Autodesk Inventor part; units mm, degrees
ref_plane "Work Plane1" through (0, -4, 0) normal (1, 0, 0) x (0, 0, -1)
ref_plane "YZ Plane" through (0, 0, 0) normal (1, 0, 0) x (0, 1, 0)
ref_plane "XZ Plane" through (0, 0, 0) normal (0, 1, 0) x (-1, 0, 0)
sketch "Sketch1" plane through (0, 0, 0) normal (0, 0, 1) x (1, 0, 0)
  line L0 (-15, -4) -> (15, -4)
  line L1 (15, -4) -> (15, 4)
  line L2 (15, 4) -> (-15, 4)
  line L3 (-15, 4) -> (-15, -4)
  line L4 (-15, -4) -> (15, 4) construction
  line L5 (15, -4) -> (-15, 4) construction
  point P0 (0, 0)
  dimension "d2" = 30
  dimension "d3" = 8
extrude "Extrusion1" add sketch "Sketch1" against normal blind 40
sketch "Sketch2" plane through (0, 0, 0) normal (0, 0, 1) x (1, 0, 0)
  circle A0 centre (0, 1.5) radius 2.75
  line L0 (-15, -4) -> (15, -4)
  point P0 (0, 0)
  point P1 (-9, -4)
  point P2 (9, -4)
  dimension "d7" = 5.5
  dimension "d8" = 5.5
extrude "Extrusion2" cut sketch "Sketch2" against normal blind 40
sketch "Sketch3" plane through (15, 4, 0) normal (0, 1, 0) x (1, 0, 0)
  circle A0 centre (-6, 8) radius 2
  line L0 (0, 0) -> (0, 40)
  line L1 (0, 0) -> (-13.8544, 0)
  point P0 (-15, 0)
  dimension "d11" = 4
  dimension "d12" = 6
  dimension "d13" = 8
extrude "Extrusion3" cut sketch "Sketch3" against normal blind 40
pattern_linear "Rectangular Pattern1" count 2 spacing 23 along (0, 0, -1) of "Extrusion3"
ref_plane "Work Plane1" through (0, -4, 0) normal (1, 0, 0) x (0, 0, -1)
mirror "Mirror1" about plane through (0, -4, 0) normal (1, 0, 0) of "Extrusion3", "Rectangular Pattern1"
properties part number "Differential_drive_wheel"
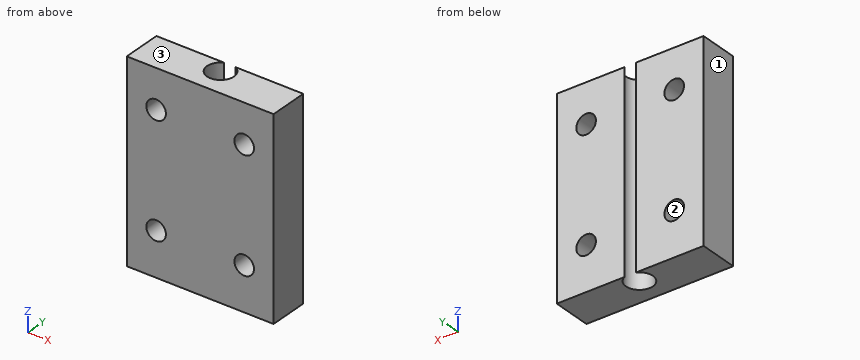
Build history of the part. All positions in model axes, mm. Face numbers are marked on the shaded views. Give positions to 0.01 mm unless a question says otherwise; leave off trailing zeros. Loops run counter-clockwise (first coordinate to the right, second up) from the corner with the lowest first, then second, coordinate; pieces in that order, holes last.
1) Band-saw the part on B-B on y = 1.5. List the corners of the cut face in (x, z).
Values follow:
outline: (-15, -40) - (-2.75, -40) - (-2.75, 0) - (-15, 0) - close; (2.75, -40) - (15, -40) - (15, 0) - (2.75, 0) - close; hole circle Ø4 at (-9, -31); hole circle Ø4 at (-9, -8); hole circle Ø4 at (9, -31); hole circle Ø4 at (9, -8)
2) Band-saw the part on D-D on z = -17. List the corners of the cut face in (x, y), then the cut area to 3 significant figures.
Values follow:
outline: (-15, -4) - (15, -4) - (15, 4) - (1.15, 4) arc R2.75 cw (long way) to (-1.15, 4) - (-15, 4) - close
area: 217 mm2
3) Band-saw the part on C-C on z = -31. List the corners of the cut face in (x, y), then the cut area to 3 significant figures.
Values follow:
outline: (-15, -4) - (-11, -4) - (-11, 4) - (-15, 4) - close; (-7, -4) - (7, -4) - (7, 4) - (1.15, 4) arc R2.75 cw (long way) to (-1.15, 4) - (-7, 4) - close; (11, -4) - (15, -4) - (15, 4) - (11, 4) - close
area: 153 mm2
4) Drop flat-ended pins along their axis: P1, Ø2.5, axis at x = -9, z = -8, coming from the +Y side; P2, Ø5, axis at x = 9, z = -8, coming from the -Y side. Give the stop position or say it passes through.
Values follow:
P1: passes through
P2: stops at y = -4
5) Band-saw the part on A-A on x = -9. List the corners of the cut face in (y, z).
Values follow:
outline: (-4, -40) - (4, -40) - (4, -33) - (-4, -33) - close; (-4, -29) - (4, -29) - (4, -10) - (-4, -10) - close; (-4, -6) - (4, -6) - (4, 0) - (-4, 0) - close
6) Probe line 1 along X through (y, z) = (-2.5, -8); line 2 along Z through (x, y) = (-9, 2.25); line 3 along X through (y, z) = (1.5, -27.5). List the from-to ranges inside material, lowest first.
Values follow:
line 1: x = -15 to -11, -7 to 7, 11 to 15
line 2: z = -40 to -33, -29 to -10, -6 to 0
line 3: x = -15 to -2.75, 2.75 to 15
7) Two-plate mould, pull along X, no slides. Class the marked faces 1, 2 and 3: released by +X, released by -X, zero draft, split by the parting line, or undercut.
Values follow:
face 1: released by -X
face 2: undercut
face 3: zero draft
